```python
from build123d import *

# Parameters (mm, degrees)
CYLINDER_R              = 2.2
CYLINDER_DEPTH          = 7
CYLINDER_PITCH_ANGLE    = 90
BOX_W                   = 8
BOX_H                   = 8
BOX_DEPTH               = 4.4
CYLINDER001_R           = 2.2
CYLINDER001_DEPTH       = 7
CYLINDER001_PITCH_ANGLE = 90


with BuildPart() as obj1:
    # Cylinder → Cylinder (new body)
    with BuildSketch(Plane.XY):
        Circle(CYLINDER_R)
    extrude(amount=CYLINDER_DEPTH)


with BuildPart() as obj1_1:
    # Cylinder pitch: moved
    add(obj1.part.rotate(Axis((0, 0, 0), (0, 1, 0)), CYLINDER_PITCH_ANGLE))


with BuildPart() as obj1_2:
    # Cylinder placement: moved
    add(obj1_1.part.moved(Location((-6, 25, -41))))


with BuildPart() as krychle:
    # Box → Box (new body)
    with BuildSketch(Plane(origin=(-7, 17, -43.3), x_dir=(1, 0, 0), z_dir=(0, 0, 1))):
        with Locations((4, 4)):
            Rectangle(BOX_W, BOX_H)
    extrude(amount=BOX_DEPTH)


with BuildPart() as fusion001003:
    # Cylinder001 → Cylinder001 (new body)
    with BuildSketch(Plane.XY):
        Circle(CYLINDER001_R)
    extrude(amount=CYLINDER001_DEPTH)


with BuildPart() as fusion001003_1:
    # Cylinder001 pitch: moved
    add(fusion001003.part.rotate(Axis((0, 0, 0), (0, 1, 0)), CYLINDER001_PITCH_ANGLE))


with BuildPart() as fusion001003_2:
    # Cylinder001 placement: moved
    add(fusion001003_1.part.moved(Location((-6, 17, -41))))

    # Fusion001003: union obj1, Krychle
    add(obj1_2.part)
    add(krychle.part)


solid = fusion001003_2.part
```
CAD build for the part. Positions are in the model's coordinates, mm. Give positions to 0.01 mm unless a question says otherwise; leave off trailing zeros. Order: outer loops, then holes, each group sorted by start corner. A loop starts at its lowest first (then second) coordinate and runs counter-clockwise, first axis right, second up. Notation, with made-up numbers: M -30.75,14.25 L -15.75,14.25 A23 ccw -15.75,48.25 Z; hole C 23,22 d7. An arc over 180 degrees is marked long. Put each result on its own line as item: value. Start each with the question number.
(1) Drill centre lines: line 1 along X through (y, z) = (26.5, -41.4); line 2 along Z through (x, y) = (-5.5, 21.25); line 3 along Y through (x, z) = (-6.5, -40.45). Where is each one in solid material? Low to high.
(2) Saw through at A-A, the plane z = -41. Write the cut outline in (x, y), then the cut area to 3 significant figures.
(3) Saw through at D-D, the plane z = -42.75. Write the cut outline in (x, y).
(4) Flat gauge pins, fed straight in: pin 1 Ø1.4 at (y, z) = (25.5, -42) entering from -X; pin 2 Ø1.3 at (x, z) = (-3, -42) entering from +Y; pin 3 Ø1.5 at (x, z) = (-4, -42.5) entering from -Y. Where does each tip first touch, or does it go through?
(5) Saw through at C-C, the plane y = 18.25. Write the cut outline in (x, z).
(6) Saw through at B-B, the plane x = -1.75. Write the cut outline in (y, z), then the cut area to 3 significant figures.
(7) Mould opens along Y. For faces 1 (the flat face through (-3, 21, -38.9)), 2 (the flat face through (-6.3, 17, -41.6)), 3 (the flat face through (1, 21, -41)), 4 (the flat face through (-6.3, 25, -41.6)) say: +Y half, -Y half, draft (parallel to the pull), parting line (faces both ways), or undercut.
Check result:
1. line 1: x = -6 to 1
1. line 2: z = -43.3 to -38.9
1. line 3: y = 17 to 25
2. outline: M -7,17 L -6,17 L -6,14.8 L 1,14.8 L 1,27.2 L -6,27.2 L -6,25 L -7,25 Z
2. area: 94.8 mm2
3. outline: M -7,17 L -6,17 L -6,15.67 L 1,15.67 L 1,26.33 L -6,26.33 L -6,25 L -7,25 Z
4. pin 1: stops at x = -7
4. pin 2: stops at y = 27.17
4. pin 3: stops at y = 14.93
5. outline: M -7,-43.3 L 1,-43.3 L 1,-38.9 L -7,-38.9 Z
6. outline: M 17,-43.3 L 25,-43.3 L 25,-43.2 A2.2 ccw long 24.34,-38.9 L 17.66,-38.9 A2.2 ccw long 17,-43.2 Z
6. area: 50.5 mm2
7. face 1: undercut
7. face 2: -Y half
7. face 3: draft
7. face 4: +Y half
